CAD build for the part. Positions are in the model's coordinates, mm. Face numbers are marked on the shaded views. A direction names the side the tool comes from. Round coordinates to 2 decimals unless told otherwise and drop trailing zeros. Write each loop counter-clockwise with the first axis right and the second up, starting at its lowest first coordinate (ties: lowest second). Pieces come first, ordered by that corner, then holes. Notation, with made-up numbers: M -28,60.25 L 22,60.25 A9 cw 22,71.25 Z; hole C 54.25,22 d1. An arc over 180 degrees is marked long. Write each question's results on one line, items separated by ' | '. Start each with the question number.
```python
from build123d import *

# Parameters (mm, degrees)
F2_SIZE  = 0.508
F4_DEPTH = 3.175
F5_COUNT = 2
F5_ANGLE = 90


with BuildPart() as f1:
    # F0 (on Top) → F1 (revolve)
    with BuildSketch(Plane.XY):
        Polygon((14.9375, 6.35), (0, 6.35), (0, 3.175), (4.7625, 3.175), (4.7625, 2.159), (7.9375, 2.159), (14.9375, 3.96875), align=None)
    revolve(axis=Axis((21.9021170629, 0, 0), (1, 0, 0)))

    # F2
    f2_edges = [f1.edges().sort_by_distance(p)[0] for p in [
        (0, -3.175, 0),
    ]]
    chamfer(f2_edges, length=F2_SIZE)



with BuildPart() as f4:
    # F3 (on Top) → F4 (new body, symmetric)
    with BuildSketch(Plane.XY):
        Polygon((6.35, 0.396875), (4.7625, 0), (6.35, -0.396875), (7.9375, -0.396875), (7.9375, 0.396875), align=None)
    extrude(amount=F4_DEPTH, both=True)


with BuildPart() as f1_1:
    add(f1.part)

    add(f4.part)  # F5 merges F4
    # F5: F4 ×2 about axis
    f5_axis = Axis((4.7625, 0, 0), (1, 0, 0))
    for i in range(1, F5_COUNT):
        add(f4.part.rotate(f5_axis, i * F5_ANGLE / (F5_COUNT - 1)))


solid = f1_1.part
```
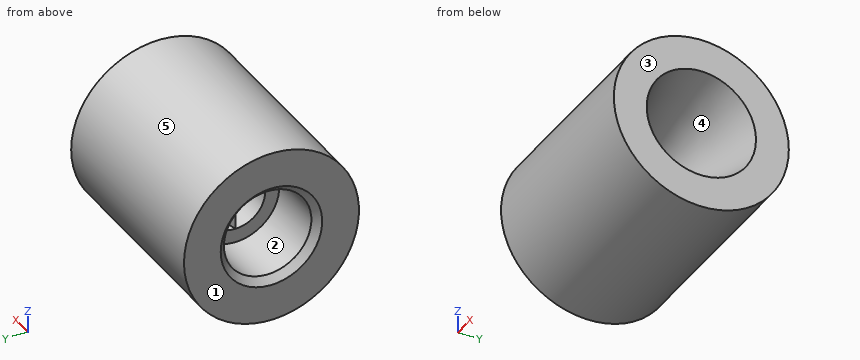
1) Wall check: line 1 along Z through (x, y) = (2.5, 0) (3 decimals); line 2 along Y through (x, z) = (7.5, 1); line 3 along Z through (x, y) = (6.5, -1.25). Give the ranges that are in metal, low to high. Write a range as from..to.
2) 3-axis set-ups, long thin cutter, end or side, ignore diameter. For the marked faces 1 and 2: which of +Z, -Z, +X, -X, +Y, -Y reach the whole face in a straight line?
3) Saw through at A-A, the plane x = 2.5. Write the cut outline in (y, z) (3 decimals).
4) Saw through at C-C, the plane z = 4.5. Write the cut outline in (x, y), plus the area to 3 significant figures.
5) Saw through at B-B, the plane z = -0.75. State how many separate pieces and enclosed holes the cut face has, plus the area to 3 significant figures.
6) Pull direction Z, two halves, no side cores. Call the marked faces 3, 4 and 5: pulls with the +Z half, pulls with the -Z half, needs draft (parallel to the pull), parting line crosses it, or undercut.
7) Saw through at D-D, the plane y = 5.5. Write the cut outline in (x, z), plus the area to 3 significant figures.
8) Drop flat-ended pins along their axis: pin 1 Ø2 at (y, z) = (-0.5, -1) entering from +X; pin 2 Ø0.5 at (x, y) = (7, -1.5) entering from +Z; pin 3 Ø3 at (x, z) = (6.5, -4) entering from -Y. Give the stop position or say it passes through.
Filled sheet:
1) line 1: z = -6.35..-3.175, 3.175..6.35 | line 2: y = -6.27..-1.91, -0.4..0.4, 1.91..6.27 | line 3: z = -6.23..-1.76, -0.4..0.4, 1.76..6.23
2) face 1: +Z, -Z, -X, +Y, -Y | face 2: -X
3) outline: C 0,0 d12.7; hole C 0,0 d6.35
4) outline: M 0,-4.48 L 14.94,-4.48 L 14.94,4.48 L 0,4.48 Z | area: 134 mm^2
5) separate pieces: 3 | enclosed holes: 0 | area: 106 mm^2
6) face 3: needs draft | face 4: undercut | face 5: parting line crosses it
7) outline: M 0,-3.17 L 14.94,-3.17 L 14.94,3.17 L 0,3.17 Z | area: 94.8 mm^2
8) pin 1: stops at x = 7.94 | pin 2: stops at z = 6.23 | pin 3: stops at y = -5.84
